Input: dimensioned drawing with shaded views. Units: mm. Origin: part minimum x, y, z. A direction names the side the tool comes from. Round coordinates to 2 decimals unless told otherwise and drop trailing zeros. Loops run counter-clockwise (first coordinate to the right, second up) from the corner with the lowest first, then second, coordinate; pieces in that order, holes last. Notation, with made-up numbers: (63.5, 34.5) -> (98.5, 34.5) arc R28 ccw to (98.5, 70.5) -> close; hole circle Ø5 at (-38.75, 19.25). An arc over 180 degrees is marked (long way). Answer as a JSON object with one key per item and string values.
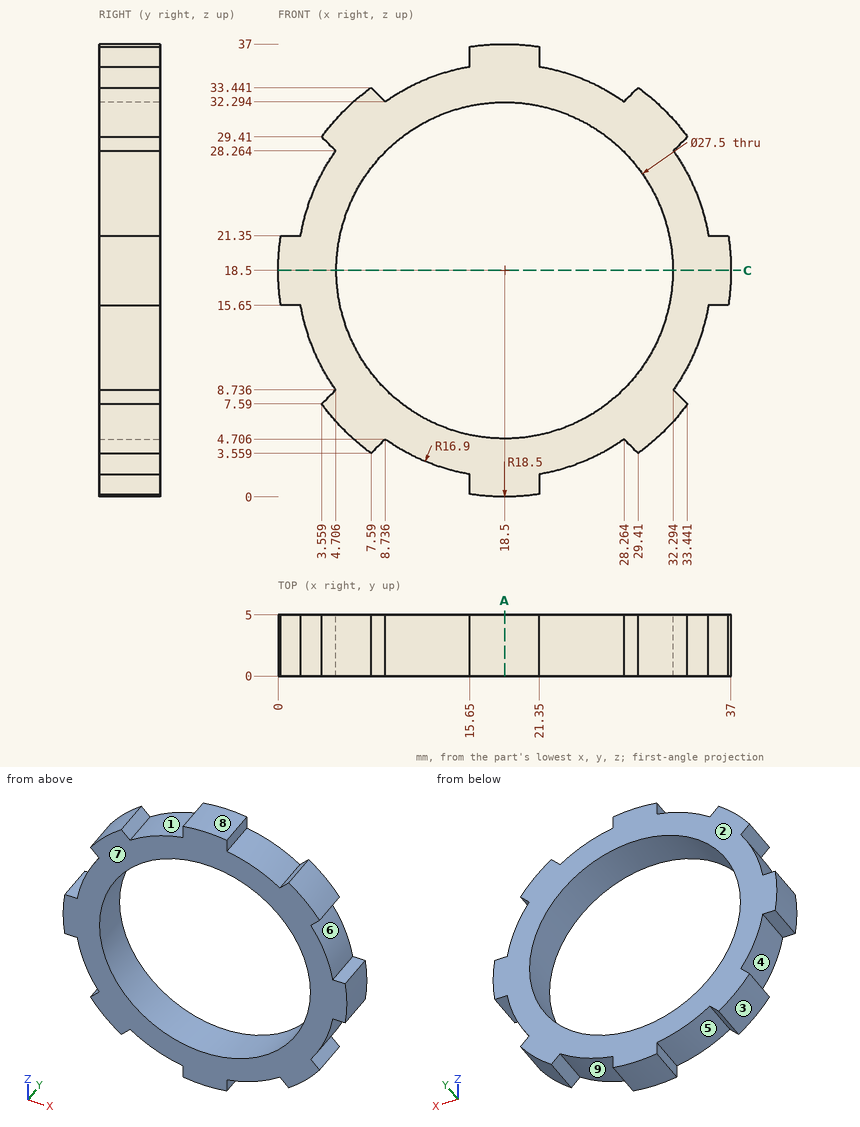
1) Draft query along Z for the marked faces 6, 7, 8 and 9. Return one class per face: +Z half, -Z half, draft (parallel to the pull), parting line (faces both ways), or undercut.
Output:
{"face 6": "undercut", "face 7": "draft", "face 8": "+Z half", "face 9": "-Z half"}
2) Section C-C, the plane z = 18.5. Output: boundary loops of the cut face in (x, y), plus the area to 3 significant figures.
Output:
{"outline": "(0, 0) -> (4.75, 0) -> (4.75, 5) -> (0, 5) -> close; (32.25, 0) -> (37, 0) -> (37, 5) -> (32.25, 5) -> close", "area": "47.5 mm^2"}
3) Ray query, probe 1 along Z at (x, y) = (18.5, 2.25); probe 2 along Z at (x, y) = (33, 4.05); probe 3 along Z at (x, y) = (4.5, 3.4) (1 decimal). Return the intervals inside material, ascending.
Output:
{"probe 1": "z = 0 to 4.75, 32.25 to 37", "probe 2": "z = 7.01 to 8.03, 9.82 to 27.18, 28.97 to 29.99", "probe 3": "z = 6.4 to 8.5, 9 to 28, 28.5 to 30.6"}
4) Contact query for flat-ended pins moving along their axis: P1, Ø2, axis at y = 2.5, z = 24.5, coming from the -X side; P2, Ø1.5, axis at y = 1.5, z = 17, coming from the -X side (1 decimal); P3, Ø1.3, axis at x = 36.5, y = 2.5, coming from the -Z side. Output: stop coordinate, or through.
Output:
{"P1": "stops at x = 2.36", "P2": "stops at x = 0", "P3": "stops at z = 15.65"}
5) Section A-A, the plane x = 18.5. Output: boundary loops of the cut face in (y, z), plus the area to 3 significant figures.
Output:
{"outline": "(0, 0) -> (5, 0) -> (5, 4.75) -> (0, 4.75) -> close; (0, 32.25) -> (5, 32.25) -> (5, 37) -> (0, 37) -> close", "area": "47.5 mm^2"}
6) Reachability of the marked faces 1, 2, 3, 4 and 5 from +Z, -Z, +X, -X, +Y, -Y: full face, straight path, thin tool, end or side. Return the list, or none.
Output:
{"face 1": "+Z, +Y, -Y", "face 2": "+Z, -Z, +X, -X, +Y", "face 3": "-Z, -X, +Y, -Y", "face 4": "-X, +Y, -Y", "face 5": "-Z, +Y, -Y"}
